Check sheet for the modelled part. Datum: model origin and axes. Units: mm. Face numbers are marked on the shaded views. Give positions to 0.01 mm unless a question says otherwise; leave off trailing zeros. Order: outer loops, then holes, each group sorted by start corner. A loop starts at its lowest first (then second) coordinate and runs counter-clockwise, first axis right, second up.
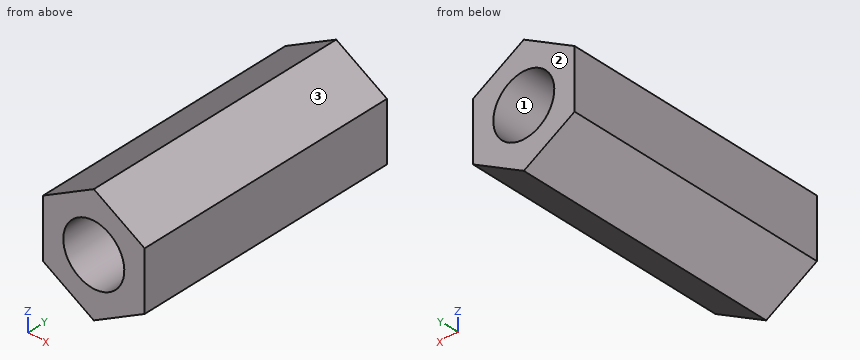
```python
from build123d import *

# Parameters (mm, degrees)
EXTRUDE_1_DEPTH     = 13
CUT_EXTRUDE_1_REACH = 15.549
SKETCH_2_R          = 1.5


with BuildPart() as part:
    # 草圖1 → 填料-伸長1 (new body)
    with BuildSketch(Plane(origin=(0, 0, 0), x_dir=(1, 0, 0), z_dir=(0, 1, 0))):
        Polygon((0, 2.886751346), (-2.5, 1.443375673), (-2.5, -1.443375673), (0, -2.886751346), (2.5, -1.443375673), (2.5, 1.443375673), align=None)
    extrude(amount=EXTRUDE_1_DEPTH)

    # 草圖2 → 除料-伸長1 (cut, up to next)
    with BuildSketch(Plane(origin=(0, 13, 0), x_dir=(-1, 0, 0), z_dir=(0, 1, 0)), mode=Mode.PRIVATE) as cut_extrude_1_sk1:
        with Locations(Location((0, 0, 0), (0, 0, 90))):
            Circle(SKETCH_2_R)
    cut_extrude_1_tool1 = extrude(cut_extrude_1_sk1.sketch, amount=-CUT_EXTRUDE_1_REACH, mode=Mode.PRIVATE) & part.part
    add(cut_extrude_1_tool1.solids().sort_by_distance((0, 13, 0))[0], mode=Mode.SUBTRACT)


solid = part.part
```
(1) Sectioned sample at A-A (z = -1.2). Enter the section's corners in (x, y), plus the area to 3 significant figures.
(2) Go/stop test with a flat-tipped pin: P1, Ø2, axis at x = 1.5, z = -0.5, coming from the -Y side. Record where the tip stops, or that it passes through.
(3) Sectioned sample at C-C (x = 0.3). Enter the section's corners in (y, z), plus the area to 3 significant figures.
(4) Sectioned sample at B-B (y = 1). Enter the section's corners in (x, z), plus the area to 3 significant figures.
(5) Sectioned sample at D-D (x = 1.9). Enter the section's corners in (y, z), plus the area to 3 significant figures.
(6) Thickness scan on L1, parallel to X at y = 3.75, z = 0; L2, parallel to X at y = 7.75, z = -1.2; L3, parallel to Z at x = -0.95, y = 12.5. Record the ranges inside material, lowest first.
(7) Release check for a two-part mould opening along X. For the marked faces 1, 2 and 3 record: released by +X, released by -X, zero draft, split by the parting line, or undercut.
Values follow:
1. outline: (-2.5, 0) - (-0.9, 0) - (-0.9, 13) - (-2.5, 13) - close; (0.9, 0) - (2.5, 0) - (2.5, 13) - (0.9, 13) - close
1. area: 41.6 mm2
2. P1: stops at y = 0
3. outline: (0, -2.71) - (13, -2.71) - (13, -1.47) - (0, -1.47) - close; (0, 1.47) - (13, 1.47) - (13, 2.71) - (0, 2.71) - close
3. area: 32.3 mm2
4. outline: (-2.5, -1.44) - (0, -2.89) - (2.5, -1.44) - (2.5, 1.44) - (0, 2.89) - (-2.5, 1.44) - close; hole circle Ø3 at (0, 0)
4. area: 14.6 mm2
5. outline: (0, -1.79) - (13, -1.79) - (13, 1.79) - (0, 1.79) - close
5. area: 46.5 mm2
6. L1: x = -2.5 to -1.5, 1.5 to 2.5
6. L2: x = -2.5 to -0.9, 0.9 to 2.5
6. L3: z = -2.34 to -1.16, 1.16 to 2.34
7. face 1: undercut
7. face 2: zero draft
7. face 3: released by +X
